Autodesk Inventor part; units mm, degrees
ref_plane "Arbeitsebene1" through (0, 0, 32) normal (0, 0, 1) x (1, 0, 0)
ref_plane "YZ Plane" through (0, 0, 0) normal (1, 0, 0) x (0, 1, 0)
ref_plane "XZ Plane" through (0, 0, 0) normal (0, 1, 0) x (-1, 0, 0)
ref_plane "Arbeitsebene1" through (0, 0, 32) normal (0, 0, 1) x (1, 0, 0)
sketch "Skizze1" plane through (0, 0, 32) normal (0, 0, 1) x (1, 0, 0)
  line L0 (0, -2) -> (-10.2, -2) construction
  line L1 (0, 0) -> (-10.2, 0) construction
  line L2 (0, 0) -> (0, -2) construction
  line L3 (-10.2, 0) -> (-10.2, -2) construction
  line L4 (-10.2, -2) -> (-0.1, -2)
  line L5 (-0.1, -2) -> (-0.1, 8)
  line L6 (-0.1, 8) -> (-10.2, 8)
  line L7 (-10.2, 8) -> (-10.2, -2)
  dimension "d0" = 10.1
  dimension "d1" = 10
extrude "Extrusion1" add sketch "Skizze1" along normal blind 5
sketch "Skizze2" plane through (-0.1, -2, 32) normal (1, 0, 0) x (0, 0, -1)
  line L0 (-3.3973, 7.8087) -> (-3.7161, 9.6721)
  line L1 (-3.0763, 5.9578) -> (-2.8181, 4.4664)
  line L2 (-2.7379, 2.2485) -> (-2.2681, 1.397) construction
  line L3 (-1.7937, 0.8596) -> (-2.122, 0.4) construction
  line L4 (-2.7257, 0.0358) -> (-1.7762, -0.6392) construction
  line L5 (0, 0) -> (0, 10) construction
  line L6 (0, 10) -> (-5, 10) construction
  line L7 (-5, 0) -> (-5, 10) construction
  line L8 (0, 0) -> (-5, 0) construction
  line L9 (0, 10) -> (-5, 10) construction
  line L10 (-3.7764, 10) -> (-2.1928, 1.2606)
  line L11 (-1.7937, 0.8596) -> (-2.122, 0.4)
  line L12 (-2.6421, 0.9776) -> (-2.2681, 1.397) construction
  line L13 (-2.122, 0.4) -> (-2.1571, -0.2183) construction
  line L14 (-1.7937, 0.8596) -> (-2.122, 0.4)
  line L15 (-1.7937, 0.8596) -> (-2.122, 0.4)
  arc A0 (-2.1928, 1.2606) -> (0, 0) centre (0, 2.5375) ccw
  line L16 (-3.7764, 10) -> (0, 10)
  line L17 (0, 10) -> (0, 0)
  point P0 (32, 2)
  point P1 (0.0012, 1.774)
extrude "Extrusion2" cut sketch "Skizze2" against normal through all
sketch "Skizze3" plane through (-10.2, -2, 37) normal (0, -1, 0) x (1, 0, 0)
  line L0 (10.2, -37) -> (0, -37) construction
  line L1 (10.2, -42) -> (10.2, -37) construction
  line L2 (0, -37) -> (0, -42) construction
  line L3 (0, -5) -> (10.1, -5) construction
  line L4 (10.1, -5) -> (10.1, 0) construction
  line L5 (0, 0) -> (10.1, 0) construction
  line L6 (0, -5) -> (0, 0) construction
  line L7 (1.0755, -3.8674) -> (-2.3192, -4.631) construction
  line L8 (4.494, -3.2233) -> (1.0755, -3.8674) construction
  line L9 (11.3855, -2.2621) -> (4.494, -3.2233) construction
  line L10 (0, -5) -> (0, 0)
  line L11 (0, -4.1093) -> (10.2, -2.4274) construction
  line L12 (10.1, -5) -> (10.1, 0)
  line L13 (10.1, 0) -> (0, 0)
  line L14 (0, 0) -> (0, 1.7809)
  line L15 (0, 0) -> (10.1, 0)
  line L16 (10.1, 0) -> (0, 1.7809)
  line L17 (10.1, 0) -> (20.3558, 0) construction
extrude "Extrusion3" add sketch "Skizze3" against normal up to surface (10 mm away)
properties part number "palm_side_plate"
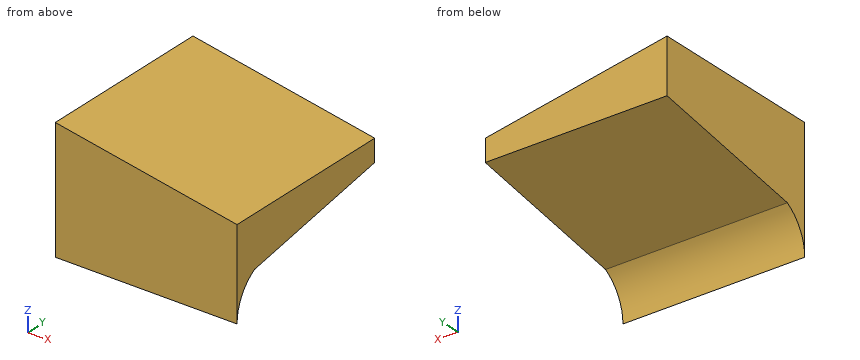
Read the model definition and answer for the solid it produces. Units are mm, in the model's axes. Round coordinates to 2 decimals unless told otherwise and drop trailing zeros. Write each loop counter-clockwise with the first axis right and the second up, starting at its lowest first coordinate (ties: lowest second). Pieces come first, ordered by that corner, then holes. Notation, with made-up numbers: M -27,-24 L 24,-24 A17 ccw 24,-4 Z; hole C 44,3.25 d9. An arc over 180 degrees is marked long. One line per item, written item: value.
Q1. Find section C-C on z = 38.25. Write down the section's boundary in (x, y), plus the area to 3 significant figures.
Data:
outline: M -10.2,-2 L -7.19,-2 L -7.19,8 L -10.2,8 Z
area: 30.1 mm2
Q2. Find section D-D on x = -9.25. Write down the section's boundary in (y, z), plus the area to 3 significant figures.
Data:
outline: M -2,32 A2.54 cw -0.74,34.19 L 8,35.78 L 8,38.61 L -2,38.61 Z
area: 38.1 mm2
Q3. Find section B-B on y = -1.5. Write down the section's boundary in (x, z).
Data:
outline: M -10.2,33.51 L -0.1,33.51 L -0.1,37 L -10.2,38.78 Z
Q4. Straight lines are drawn through the part: line 1 (Z direction, x = -9.25, y = 4.5); line 2 (Z direction, x = -5, y = 3.75); line 3 (Y direction, x = -5.75, z = 34). For each, find the intervals that lie inside material, in ascending order. Write a range as [from, to].
Data:
line 1: [35.14, 38.61]
line 2: [35.01, 37.86]
line 3: [-2, -1.02]
Q5. Find section A-A on x = -6.25. Write down the section's boundary in (y, z).
Data:
outline: M -2,32 A2.54 cw -0.74,34.19 L 8,35.78 L 8,38.08 L -2,38.08 Z
